Could you check a few things on this model? Use its own coordinates, in mm. Face numbers are marked on the shaded views. A direction names the side the tool comes from. Give positions to 0.01 mm unless a question says otherwise; leave off trailing zeros. Loops run counter-clockwise (first coordinate to the right, second up) from the corner with the lowest first, then second, coordinate; pieces in that order, holes last. Notation, with made-up numbers: (71.25, 39) - (104.25, 39) arc R22 ccw to (104.25, 68) - close; hole circle Ø8 at (84, 26). An arc over 180 degrees is marked (long way). Use CSV: the item, a comma, the result in double quotes.
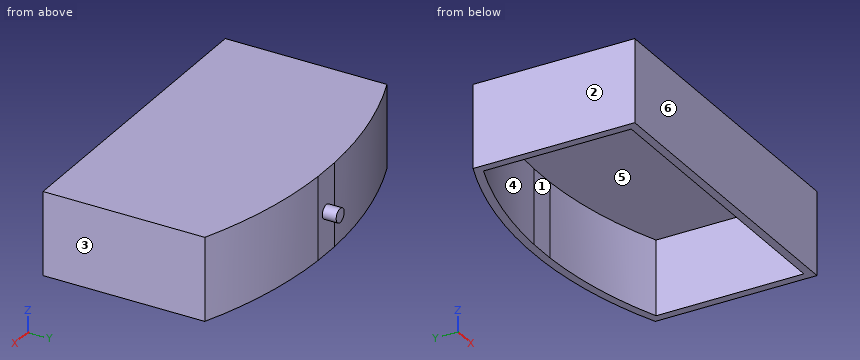
from build123d import *

# Parameters (mm, degrees)
BOSS_EXTRUDE1_DEPTH = 30
CUT_EXTRUDE1_DEPTH  = 27
SKETCH3_R           = 2.5
BOSS_EXTRUDE2_DEPTH = 5


with BuildPart() as part:
    # Sketch1 → Boss-Extrude1 (new body)
    with BuildSketch(Plane.XY):
        with BuildLine():
            Line((-5, 149.916643506), (5, 149.916643506))
            ThreePointArc((5, 149.916643506), (31.23486102, 146.711906324), (56.5, 138.952329955))
            Line((56.5, 138.952329955), (56.5, 80.652329955))
            Line((56.5, 80.652329955), (-56.5, 80.652329955))
            Line((-56.5, 80.652329955), (-56.5, 138.952329955))
            ThreePointArc((-56.5, 138.952329955), (-31.23486102, 146.711906324), (-5, 149.916643506))
        make_face()
    extrude(amount=BOSS_EXTRUDE1_DEPTH)

    # Sketch2 → Cut-Extrude1 (cut)
    with BuildSketch(Plane(origin=(0, 0, 0), x_dir=(-1, 0, 0), z_dir=(0, 0, -1))):
        with BuildLine():
            Line((4.949733431, 146.916643506), (-4.949733431, 146.916643506))
            ThreePointArc((-4.949733431, 146.916643506), (-29.649320321, 143.978879717), (-53.5, 136.91877154))
            Line((-53.5, 136.91877154), (-53.5, 83.652329955))
            Line((-53.5, 83.652329955), (53.5, 83.652329955))
            Line((53.5, 83.652329955), (53.5, 136.91877154))
            ThreePointArc((53.5, 136.91877154), (29.649320321, 143.978879717), (4.949733431, 146.916643506))
        make_face()
    extrude(amount=-CUT_EXTRUDE1_DEPTH, mode=Mode.SUBTRACT)

    # Sketch3 → Boss-Extrude2 (add)
    with BuildSketch(Plane(origin=(0, 149.916643506, 0), x_dir=(1, 0, 0), z_dir=(0, 1, 0))):
        with Locations(Location((0, -15, 0), (0, 0, 270))):
            Circle(SKETCH3_R)
    extrude(amount=BOSS_EXTRUDE2_DEPTH)


solid = part.part
1) We'd pull the mould along X, two halves only. Please class the marked faces 3, 4, 5 and 6: +X half, -X half, draft (parallel to the pull), parting line (faces both ways), or undercut.
Answer below:
face 3,"+X half"
face 4,"undercut"
face 5,"undercut"
face 6,"draft"
2) Suppose I cut it at D-D (z = 15). Please give me the cut outline in (x, y), plus the area to 3 significant figures.
Answer below:
outline,"(-56.5, 80.65) - (56.5, 80.65) - (56.5, 138.95) arc R150 ccw to (5, 149.92) - (2.5, 149.92) - (2.5, 154.92) - (-2.5, 154.92) - (-2.5, 149.92) - (-5, 149.92) arc R150 ccw to (-56.5, 138.95) - close; hole (-53.5, 83.65) - (53.5, 83.65) - (53.5, 136.92) arc R147 ccw to (4.95, 146.92) - (-4.95, 146.92) arc R147 ccw to (-53.5, 136.92) - close"
area,"1,030 mm2"
3) I need wall thicknesses on line 1 along X through (y, z) = (86, 21.5); line 2 along Y through (x, z) = (3.5, 11.75); line 3 along Z through (x, y) = (29, 126.5). Which ranges of each line are inside material? Lowest first, please.
Answer below:
line 1,"x = -56.5 to -53.5, 53.5 to 56.5"
line 2,"y = 80.65 to 83.65, 146.92 to 149.92"
line 3,"z = 27 to 30"
4) Suppose I cut it at A-A (z = 6.75). Please give me the cut outline in (x, y).
Answer below:
outline,"(-56.5, 80.65) - (56.5, 80.65) - (56.5, 138.95) arc R150 ccw to (5, 149.92) - (-5, 149.92) arc R150 ccw to (-56.5, 138.95) - close; hole (-53.5, 83.65) - (53.5, 83.65) - (53.5, 136.92) arc R147 ccw to (4.95, 146.92) - (-4.95, 146.92) arc R147 ccw to (-53.5, 136.92) - close"
5) I'm going to push flat-ended pins straight in: P1, Ø6, axis at x = 43, z = 26, coming from the +Y side; P2, Ø12, axis at x = -45, z = 9.5, coming from the +Y side; P3, Ø3, axis at x = -4.5, z = 8.5, coming from the +Y side. Where does each tip first touch, or does it pass through?
Answer below:
P1,"stops at y = 144.57"
P2,"stops at y = 144.84"
P3,"stops at y = 149.92"
6) Suppose I cut it at C-C (x = 0). Please give me the cut outline in (y, z), plus the area to 3 significant figures.
Answer below:
outline,"(80.65, 0) - (83.65, 0) - (83.65, 27) - (146.92, 27) - (146.92, 0) - (149.92, 0) - (149.92, 12.5) - (154.92, 12.5) - (154.92, 17.5) - (149.92, 17.5) - (149.92, 30) - (80.65, 30) - close"
area,"395 mm2"
7) Suppose I cut it at B-B (y = 94.5). Please give me the cut outline in (x, z).
Answer below:
outline,"(-56.5, 0) - (-53.5, 0) - (-53.5, 27) - (53.5, 27) - (53.5, 0) - (56.5, 0) - (56.5, 30) - (-56.5, 30) - close"
8) Which directions (+Z, -Z, +X, -X, +Y, -Y) give clear straight access to the entire face, cutting with the end or side of a thin tool? Please do the marked faces 1 and 2.
Answer below:
face 1,"-Z"
face 2,"+Z, -Z, -X, +Y, -Y"
